Verification items for the finished model (mm, model axes). Coordinates: 2 decimals unless noted, no trailing zeros. Answer as CSV lines item,"result".
```python
from build123d import *

# Parameters (mm, degrees)
SKETCH_1_R          = 11.5
SKETCH_1_R_2        = 5.5
SKETCH_1_R_3        = 1
EXTRUDE_1_DEPTH     = 2.5
EXTRUDE_START       = -1.3
SKETCH_2_R          = 5.5
EXTRUDE_2_DEPTH     = 1.3
SKETCH_5_R          = 2.5
CUT_EXTRUDE_1_DEPTH = 1
SKETCH_6_R          = 2
EXTRUDE_3_DEPTH     = 7.5
SKETCH_7_R          = 3
EXTRUDE_4_DEPTH     = 4
SKETCH_10_R         = 1
EXTRUDE_5_DEPTH     = 2
CHAMFER_1_SIZE      = 0.3
SKETCH_11_R         = 2.300425052
EXTRUDE_6_DEPTH     = 1.5
CHAMFER_2_SIZE      = 1
CHAMFER_3_SIZE      = 0.5
CHAMFER_4_SIZE      = 0.5


with BuildPart() as part:
    # 草图1 → 凸台-拉伸1 (new body)
    with BuildSketch(Plane(origin=(1.966710395, 32.715392416, 1.10826425), x_dir=(0.9981999912017503, -0.059938758009620605, -0.002030480999629514), z_dir=(-0.05997314036154614, -0.9976277272985652, -0.03379556421002548))):
        with Locations(Location((-129.040965006, -30.648001563, 0), (0, 0, 0.116404566))):
            Circle(SKETCH_1_R)
        with Locations(Location((-129.040965006, -30.648001563, 0), (0, 0, 0.116404566))):
            Circle(SKETCH_1_R_2, mode=Mode.SUBTRACT)
        with Locations(Location((-135.609495823, -34.813863168, 0), (0, 0, 0.116404566))):
            Circle(SKETCH_1_R_3, mode=Mode.SUBTRACT)
        with Locations(Location((-133.206826611, -24.079470746, 0), (0, 0, 0.116404566))):
            Circle(SKETCH_1_R_3, mode=Mode.SUBTRACT)
        with Locations(Location((-122.472434189, -26.482139959, 0), (0, 0, 0.116404566))):
            Circle(SKETCH_1_R_3, mode=Mode.SUBTRACT)
        with Locations(Location((-124.875103402, -37.21653238, 0), (0, 0, 0.116404566))):
            Circle(SKETCH_1_R_3, mode=Mode.SUBTRACT)
    extrude(amount=EXTRUDE_1_DEPTH)

    # 草图2 → 凸台-拉伸2 (add)
    with BuildSketch(Plane(origin=(1.816777544, 30.221323097, 1.02377534), x_dir=(0.9981999912017503, -0.059938758009620605, -0.002030480999629515), z_dir=(-0.05997314036154614, -0.9976277272985652, -0.03379556421002549)).offset(EXTRUDE_START)):
        with Locations(Location((-129.040965006, -30.648001563, 0), (0, 0, 0.116404566))):
            Circle(SKETCH_2_R)
    extrude(amount=EXTRUDE_2_DEPTH)

    # 草图5 → 切除-拉伸1 (cut)
    with BuildSketch(Plane(origin=(1.816777544, 30.221323097, 1.02377534), x_dir=(0.9981999912017503, -0.059938758009620605, -0.002030480999629515), z_dir=(-0.05997314036154614, -0.9976277272985652, -0.03379556421002564))):
        with Locations(Location((-135.609495823, -34.813863168, 0), (0, 0, 0.116404566))):
            Circle(SKETCH_5_R)
        with Locations(Location((-133.206826611, -24.079470746, 0), (0, 0, 0.116404566))):
            Circle(SKETCH_5_R)
        with Locations(Location((-122.472434189, -26.482139959, 0), (0, 0, 0.116404566))):
            Circle(SKETCH_5_R)
        with Locations(Location((-124.875103402, -37.21653238, 0), (0, 0, 0.116404566))):
            Circle(SKETCH_5_R)
    extrude(amount=-CUT_EXTRUDE_1_DEPTH, mode=Mode.SUBTRACT)

    # 草图6 → 凸台-拉伸3 (add)
    with BuildSketch(Plane(origin=(1.816777544, 30.221323097, 1.02377534), x_dir=(0.9981999912017503, -0.059938758009620605, -0.002030480999629515), z_dir=(-0.05997314036154614, -0.9976277272985652, -0.033795564210025573))):
        with Locations(Location((-129.040965006, -29.648001563, 0), (0, 0, 180.116404566))):
            Circle(SKETCH_6_R)
    extrude(amount=EXTRUDE_3_DEPTH)

    # 草图7 → 凸台-拉伸4 (add)
    with BuildSketch(Plane(origin=(1.816777544, 30.221323097, 1.02377534), x_dir=(0.9981999912017503, -0.059938758009620605, -0.002030480999629515), z_dir=(-0.05997314036154614, -0.9976277272985652, -0.033795564210025615))):
        with Locations(Location((-129.040965006, -29.648001563, 0), (0, 0, 0.116404566))):
            Circle(SKETCH_7_R)
    extrude(amount=EXTRUDE_4_DEPTH)

    # 草图10 → 凸台-拉伸5 (add)
    with BuildSketch(Plane(origin=(1.366978991, 22.739115143, 0.770308608), x_dir=(0.9981999912017503, -0.05993875800962059, -0.002030480999629514), z_dir=(-0.05997314036154613, -0.9976277272985652, -0.03379556421002559))):
        with Locations(Location((-129.040965006, -30.648001563, 0), (0, 0, 269.999999999))):
            Circle(SKETCH_10_R)
    extrude(amount=EXTRUDE_5_DEPTH)

    # 倒角1
    # the kernel refuses this chamfer: 0.3 mm, written as the material it takes off along each edge
    with BuildSketch(Plane(origin=(-127.441711143, 31.477448067, -28.598680652), x_dir=(-1.5916157281026276e-11, 0.0338565062200545, -0.9994267041592252), z_dir=(-0.9981999912017503, 0.059938758009080766, 0.002030481015565288))) as chamfer_1_piece_1_section:
        Polygon((2, -CHAMFER_1_SIZE), (2 - CHAMFER_1_SIZE, 0), (2, 0), align=None)
    chamfer_1_piece_1 = revolve(axis=Axis((-127.441711143, 31.477448067, -28.598680652), (-0.05997314036154614, -0.9976277272985652, -0.03379556421002558)), revolution_arc=270.116404567, mode=Mode.PRIVATE)
    chamfer_1_piece_1 = chamfer_1_piece_1 - Plane(origin=(-127.43302189, 31.655846599, -29.593210861), x_dir=(-1.742146691663825e-11, 0.03385650622014407, -0.9994267041592222), z_dir=(0.05997314036154613, 0.9976277272985653, 0.033795564210025594)) * Cylinder(1, 8, mode=Mode.PRIVATE)
    add(chamfer_1_piece_1, mode=Mode.SUBTRACT)
    with BuildSketch(Plane(origin=(-127.231805152, 34.969145112, -28.480396177), x_dir=(0.9981979311307728, -0.060007418593410425, 2.631376598098256e-12), z_dir=(0.0020279845707766217, 0.033734662275686965, -0.9994287667661592))) as chamfer_1_piece_2:
        Polygon((3, -CHAMFER_1_SIZE), (3 - CHAMFER_1_SIZE, 0), (3, 0), align=None)
    revolve(axis=Axis((-127.231805152, 34.969145112, -28.480396177), (-0.05997314036154614, -0.9976277272985652, -0.03379556421002563)), mode=Mode.SUBTRACT)
    with BuildSketch(Plane(origin=(-127.561657424, 29.516049118, -29.665698484), x_dir=(-1.7422507880890286e-11, 0.03385650622014249, -0.9994267041592222), z_dir=(-0.9981999912017504, 0.05993875800902966, 0.0020304810170733417))) as chamfer_1_piece_3:
        Polygon((1, -CHAMFER_1_SIZE), (1 - CHAMFER_1_SIZE, 0), (1, 0), align=None)
    revolve(axis=Axis((-127.561657424, 29.516049118, -29.665698484), (-0.05997314036154613, -0.9976277272985653, -0.033795564210025594)), mode=Mode.SUBTRACT)
    with BuildSketch(Plane(origin=(-127.441711143, 31.477448067, -28.598680652), x_dir=(-0.9981979311307727, 0.060007418593412805, -2.629008122312364e-12), z_dir=(-0.0020279845707743367, -0.03373466227568705, 0.9994287667661592))) as chamfer_1_piece_4_section:
        Polygon((2, -CHAMFER_1_SIZE), (2 - CHAMFER_1_SIZE, 0), (2, 0), align=None)
    chamfer_1_piece_4 = revolve(axis=Axis((-127.441711143, 31.477448067, -28.598680652), (-0.05997314036154614, -0.9976277272985652, -0.03379556421002558)), revolution_arc=89.883595433, mode=Mode.PRIVATE)
    chamfer_1_piece_4 = chamfer_1_piece_4 - Plane(origin=(-127.432917992, 31.657574909, -29.593152313), x_dir=(-1.742146691663825e-11, 0.03385650622014407, -0.9994267041592222), z_dir=(0.05997314036154613, 0.9976277272985653, 0.033795564210025594)) * Cylinder(1, 9, mode=Mode.PRIVATE)
    add(chamfer_1_piece_4, mode=Mode.SUBTRACT)

    # 草图11 → 凸台-拉伸6 (add)
    with BuildSketch(Plane(origin=(1.576884982, 26.230812188, 0.888593083), x_dir=(0.9981999912017503, -0.059938758009620605, -0.0020304809996295197), z_dir=(-0.05997314036154614, -0.9976277272985652, -0.03379556421002562))):
        with Locations(Location((-129.040965006, -29.648001563, 0), (0, 0, 180.116404566))):
            Circle(SKETCH_11_R)
    extrude(amount=EXTRUDE_6_DEPTH)

    # 倒角2
    chamfer_2_edges = [part.edges().sort_by_distance(p)[0] for p in [
        (-138.471188798, 39.683597842, -29.344640624),
    ]]
    chamfer(chamfer_2_edges, length=CHAMFER_2_SIZE)

    # 倒角3
    # the kernel refuses this chamfer: 0.5 mm, written as the material it takes off along each edge
    with BuildSketch(Plane(origin=(-122.833549573, 38.966203462, -35.917864433), x_dir=(0.9981979311307727, -0.06000741859341191, 2.6318502932554117e-12), z_dir=(0.0020279845707771465, 0.03373466227568696, -0.9994287667661592))) as chamfer_3_piece_1:
        Polygon((2.5 + CHAMFER_3_SIZE, 0), (2.5, -CHAMFER_3_SIZE), (2.5, 0), align=None)
    revolve(axis=Axis((-122.833549573, 38.966203462, -35.917864433), (-0.05997314036154614, -0.9976277272985652, -0.03379556421002566)), mode=Mode.SUBTRACT)
    with BuildSketch(Plane(origin=(-120.435205187, 38.458761429, -25.194504568), x_dir=(0.9981979311307725, -0.06000741859341508, 2.6304292077839058e-12), z_dir=(0.002027984570775836, 0.033734662275687034, -0.9994287667661591))) as chamfer_3_piece_2:
        Polygon((2.5 + CHAMFER_3_SIZE, 0), (2.5, -CHAMFER_3_SIZE), (2.5, 0), align=None)
    revolve(axis=Axis((-120.435205187, 38.458761429, -25.194504568), (-0.05997314036154614, -0.9976277272985652, -0.03379556421002566)), mode=Mode.SUBTRACT)
    with BuildSketch(Plane(origin=(-131.150275607, 39.020821594, -22.771416816), x_dir=(0.9981979311307727, -0.06000741859341225, 2.633271378726947e-12), z_dir=(0.0020279845707785755, 0.033734662275686875, -0.9994287667661592))) as chamfer_3_piece_3:
        Polygon((2.5 + CHAMFER_3_SIZE, 0), (2.5, -CHAMFER_3_SIZE), (2.5, 0), align=None)
    revolve(axis=Axis((-131.150275607, 39.020821594, -22.771416816), (-0.05997314036154614, -0.9976277272985652, -0.03379556421002566)), mode=Mode.SUBTRACT)
    with BuildSketch(Plane(origin=(-133.548619994, 39.528263626, -33.494776681), x_dir=(0.9981979311307727, -0.06000741859341225, 2.6318502932554267e-12), z_dir=(0.0020279845707771578, 0.03373466227568696, -0.9994287667661592))) as chamfer_3_piece_4:
        Polygon((2.5 + CHAMFER_3_SIZE, 0), (2.5, -CHAMFER_3_SIZE), (2.5, 0), align=None)
    revolve(axis=Axis((-133.548619994, 39.528263626, -33.494776681), (-0.05997314036154614, -0.9976277272985652, -0.03379556421002566)), mode=Mode.SUBTRACT)

    # 倒角4
    chamfer_4_edges = [part.edges().sort_by_distance(p)[0] for p in [
        (-132.33206836, 41.817622648, -29.260151714),
    ]]
    chamfer(chamfer_4_edges, length=CHAMFER_4_SIZE)


solid = part.part
```
Item 1: Depth check by flat-ended pin: pin 1 Ø5 at (x, y) = (-128.5, 36.5) entering from +Z; pin 2 Ø4 at (y, z) = (40, -20.5) entering from -X; pin 3 Ø1.5 at (y, z) = (38, -20.5) entering from +X. Enter the tip coordinate at first touch or a pass-through.
Answer list:
pin 1,"z = -18.63"
pin 2,"x = -136.17"
pin 3,"x = -120.2"
Item 2: Thickness scan on line 1 (Z direction, x = -132.5, y = 39.75); line 2 (Z direction, x = -127.75, y = 33.25); line 3 (Y direction, x = -121.5, z = -39). Record the ranges inside material, lowest first.
Answer list:
line 1,"-38.39 to -36.09, -31.06 to -24.83, -20.67 to -19.53"
line 2,"-30.5 to -26.58"
line 3,"39.6 to 41.5"
Item 3: Release check for a two-part mould opening along Y. For faces 1 (the cylindrical face through (-120.41, 39.54, -35.14)), 2 (the cylindrical face through (-132.52, 41.24, -33.82)), 3 (the conical face through (-128.39, 38.893, -18.762)) record: +Y half, -Y half, draft (parallel to the pull), parting line (faces both ways), or undercut.
Answer list:
face 1,"undercut"
face 2,"parting line"
face 3,"-Y half"
